Check sheet for the modelled part. Datum: model origin and axes. Units: mm. A direction names the side the tool comes from. Round coordinates to 2 decimals unless told otherwise and drop trailing zeros. Write each loop counter-clockwise with the first axis right and the second up, starting at its lowest first coordinate (ties: lowest second). Pieces come first, ordered by that corner, then holes. Notation, with made-up numbers: (2.5, -0.5) -> (31.5, -0.5) arc R28 ccw to (31.5, 34.5) -> close; hole circle Ø2 at (-21, 4). An arc over 180 degrees is marked (long way). Write item = value, one per line.
from build123d import *

# Parameters (mm, degrees)
Y_KSEKLIK_EKSTR_ZYON1_DEPTH = 700
IZIM2_W                     = 360.449824165
IZIM2_H                     = 531.81345569
KES_EKSTR_ZYON1_DEPTH       = 700
IZIM3_W                     = 260.927179237
IZIM3_H                     = 250.055213435
KES_EKSTR_ZYON2_DEPTH       = 700
IZIM4_W                     = 592.507682974
IZIM4_H                     = 203.257851284
KES_EKSTR_ZYON3_DEPTH       = 100


with BuildPart() as part:
    # Çizim1 → Yükseklik-Ekstrüzyon1 (new body)
    with BuildSketch(Plane.XY):
        with BuildLine():
            Line((210, -500), (250, -500))
            Line((250, -500), (250, 300))
            Line((250, 300), (250, 500))
            Line((250, 500), (-181.095158938, 500))
            ThreePointArc((-181.095158938, 500), (-229.338190574, 451.785260133), (-250, 386.784176503))
            Line((-250, 386.784176503), (-250, -480))
            ThreePointArc((-250, -480), (-244.142135624, -494.142135624), (-230, -500))
            Line((-230, -500), (-190, -500))
            ThreePointArc((-190, -500), (10, -300), (210, -500))
        make_face()
        with BuildLine():
            ThreePointArc((1180.672940492, -500), (980.672940492, -300), (780.672940492, -500))
            Line((780.672940492, -500), (250, -500))
            Line((250, -500), (250, 300))
            Line((250, 300), (1250, 300))
            Line((1250, 300), (1250, -500))
            Line((1250, -500), (1180.672940492, -500))
        make_face()
    extrude(amount=-Y_KSEKLIK_EKSTR_ZYON1_DEPTH)

    # Çizim2 → Kes-Ekstrüzyon1 (cut)
    with BuildSketch(Plane(origin=(1250, 0, 0), x_dir=(0, 0, -1), z_dir=(1, 0, 0))):
        with Locations((343.970170228, 34.093272155)):
            Rectangle(IZIM2_W, IZIM2_H)
    extrude(amount=-KES_EKSTR_ZYON1_DEPTH, mode=Mode.SUBTRACT)

    # Çizim3 → Kes-Ekstrüzyon2 (cut)
    with BuildSketch(Plane(origin=(0, 0, -700), x_dir=(-1, 0, 0), z_dir=(0, 0, -1))):
        with Locations((23.407496445, 308.297887372)):
            Rectangle(IZIM3_W, IZIM3_H)
    extrude(amount=-KES_EKSTR_ZYON2_DEPTH, mode=Mode.SUBTRACT)

    # Çizim4 → Kes-Ekstrüzyon3 (cut)
    with BuildSketch(Plane.ZY.offset(250)):
        with Locations((-349.282031692, 285.155250861)):
            Rectangle(IZIM4_W, IZIM4_H)
    extrude(amount=-KES_EKSTR_ZYON3_DEPTH, mode=Mode.SUBTRACT)


solid = part.part
(1) Release check for a two-part mould opening along Z. For faces 1 (the flat face through (905, 30, -524.195)), 2 (the flat face through (490, 7, -700)), 3 (the flat face through (-22, 183.27, -355)) record: pulls with the +Z half, pulls with the -Z half, needs draft (parallel to the pull), parting line crosses it, or undercut.
Worked answers:
face_1 = undercut
face_2 = pulls with the -Z half
face_3 = needs draft
(2) Sectioned sample at B-B on z = -610.5. Enter the section's corners in (x, y).
Worked answers:
outline = (-250, -480) arc R20 ccw to (-230, -500) -> (-190, -500) arc R200 cw to (210, -500) -> (780.67, -500) arc R200 cw to (1180.67, -500) -> (1250, -500) -> (1250, 300) -> (250, 300) -> (250, 500) -> (-181.1, 500) arc R144.08 ccw to (-250, 386.78) -> (-153.87, 386.78) -> (-153.87, 433.33) -> (107.06, 433.33) -> (107.06, 183.27) -> (-153.87, 183.27) -> (-153.87, 183.53) -> (-250, 183.53) -> close
(3) Go/stop test with flat-tipped pins: P1, Ø8, axis at y = 218, z = -327, coming from the +X side; P2, Ø1.5, axis at x = 111, z = -561, coming from the -Y side. Record where each tip stops, or that it passes through.
Worked answers:
P1 = 550
P2 = -327.82
(4) Material ranges on L1, parallel to X at y = -447, z = -653.5; L2, parallel to Z at x = 612.5, y = -75.5; L3, parallel to X at y = -320.5, z = -216, recorded low to high. Write a range as [from, to].
Worked answers:
L1 = [-250, -182.85], [202.85, 787.82], [1173.52, 1250]
L2 = [-700, -524.2], [-163.75, 0]
L3 = [-250, -78.2], [98.2, 892.47], [1068.88, 1250]
(5) Sectioned sample at C-C on y = -206. Enter the section's corners in (x, z).
Worked answers:
outline = (-250, -700) -> (1250, -700) -> (1250, -524.2) -> (550, -524.2) -> (550, -163.75) -> (1250, -163.75) -> (1250, 0) -> (-250, 0) -> close
(6) Sectioned sample at D-D on x = 572. Enter the section's corners in (y, z).
Worked answers:
outline = (-500, -700) -> (300, -700) -> (300, -524.2) -> (-231.81, -524.2) -> (-231.81, -163.75) -> (300, -163.75) -> (300, 0) -> (-500, 0) -> close
(7) Access from +Z, -Z, +X, -X, +Y, -Y to the whole of each face (thin tool, end or side, straight path). Record for faces 4 (the flat face through (905, -231.813, -341)), 5 (the flat face through (37, 500, -345)), 6 (the flat face through (-153.871, 390, -355)), 7 (the flat face through (250, 399, -345)), 8 (the flat face through (-203, 386.784, -353)).
Worked answers:
face_4 = +X, +Y
face_5 = +Z, -Z, +X, -X, +Y
face_6 = +Z, -Z
face_7 = +Z, -Z, +X, +Y
face_8 = -X
(8) Sectioned sample at A-A on x = 10. Enter the section's corners in (y, z).
Worked answers:
outline = (-300, -700) -> (183.27, -700) -> (183.27, 0) -> (-300, 0) -> close; (433.33, -700) -> (500, -700) -> (500, 0) -> (433.33, 0) -> close
